Geometry: final body of the model. Coordinates: model frame, mm. A direction names the side the tool comes from. Round coordinates to 2 decimals unless told otherwise and drop trailing zeros. Loops run counter-clockwise (first coordinate to the right, second up) from the corner with the lowest first, then second, coordinate; pieces in that order, holes last. Notation, with made-up numbers: (19.5, 32.25) - (34.5, 32.25) arc R20 ccw to (34.5, 56.25) - close; hole circle Ø8 at (59, 46.25). An arc over 180 degrees is marked (long way). Answer as a JSON object with one key per item and string values. Group by question number.
Item 1: Section C-C (y = -4). Return the cut outline in (x, z), plus the area to 3 significant figures.
Item 2: Line query: line 1 (Z direction, x = 65.75, y = -2); line 2 (X direction, y = 0, z = 28.5); line 3 (Y direction, x = 66.5, z = 9.5). Output: solid intervals per line, ascending.
Item 3: Draft query along X for faces 4 (the face through (72.08, -5.04, 14.79)), 5 (the face through (67.43, 0.45, 14.87)), 6 (the face through (66, -2.95, 26)). Return one class per face: released by +X, released by -X, zero draft, split by the parting line, or undercut.
Item 4: First-contact query: pin 1 (1.5 mm diameter, centred on x = 65, z = 19.5, fed in from -Y); pin 2 (0.8 mm diameter, centred on x = 65, z = 25.5, fed in from -Y); pin 3 (0.8 mm diameter, centred on y = 0.5, z = 25.5, fed in from -X); pin 4 (4 mm diameter, centred on x = 66, y = 0, fed in from -Z). Flat tips, straight axial feed; report the tip coordinate or a pass-through.
Item 5: Section D-D (x = 65.5). Return the cut outline in (y, z).
Item 6: Reachability of faces 1 (the face through (67.4, 1.3, 27)), 2 (the face through (71.403, 3.725, 15.21)), 3 (the face through (71, 0, 4)) from +Z, -Z, +X, -X, +Y, -Y: full face, straight path, thin tool, end or side. Return the list, or none.
Item 7: Section B-B (z = 11.5). Return the cut outline in (x, y).
Item 8: Section A-A (z = 24.75). Return the cut outline in (x, y).
```python
from build123d import *

# Parameters (mm, degrees)
SKETCH_R        = 1.5
PAD_DEPTH       = 30
POCKET_DEPTH    = 30.001
FILLET_R        = 4.5
SKETCH002_W     = 5.9
SKETCH002_H     = 2.8
POCKET001_DEPTH = 71


with BuildPart() as part:
    # Sketch → Pad (new body)
    with BuildSketch(Plane.XY):
        with BuildLine():
            Line((61.848971, 4.324901), (72.822176, 5.092223))
            ThreePointArc((72.822176, -5.092223), (73, 0), (72.822176, 5.092223))
            Line((72.822176, -5.092223), (61.848971, -4.324901))
            ThreePointArc((61.848971, -4.324901), (62, 0), (61.848971, 4.324901))
        make_face()
        with Locations((66, 0)):
            Circle(SKETCH_R, mode=Mode.SUBTRACT)
    extrude(amount=PAD_DEPTH)

    # Sketch001 (on Face7 of Pad) → Pocket (cut, through all)
    with BuildSketch(Plane.XY.offset(30)):
        with BuildLine():
            ThreePointArc((71.32583, -4.987588), (71.402012, -3.742021), (71.456444, -2.495314))
            Line((69.257784, -2.418535), (71.456444, -2.495314))
            ThreePointArc((69.131189, -4.834124), (69.205027, -3.626882), (69.257784, -2.418535))
            Line((69.131189, -4.834124), (71.32583, -4.987588))
        make_face()
        with BuildLine():
            Line((69.257784, 2.418535), (71.456444, 2.495314))
            ThreePointArc((71.456444, 2.495314), (71.402012, 3.742021), (71.32583, 4.987588))
            Line((69.131189, 4.834124), (71.32583, 4.987588))
            ThreePointArc((69.257784, 2.418535), (69.205027, 3.626882), (69.131189, 4.834124))
        make_face()
    extrude(amount=-POCKET_DEPTH, mode=Mode.SUBTRACT)

    # Fillet
    fillet_edges = [part.edges().sort_by_distance(p)[0] for p in [
        (61.848971, 4.324901, 15),
        (61.848971, -4.324901, 15),
    ]]
    fillet(fillet_edges, radius=FILLET_R)

    # Sketch002 → Pocket001 (cut)
    with BuildSketch(Plane.YZ):
        with Locations((0, 25.6)):
            Rectangle(SKETCH002_W, SKETCH002_H)
        with Locations((0, 4.4)):
            Rectangle(SKETCH002_W, SKETCH002_H)
    extrude(amount=POCKET001_DEPTH, mode=Mode.SUBTRACT)


solid = part.part
```
Values:
{
 "1": {"outline": "(64.19, 0) - (69.18, 0) - (69.18, 30) - (64.19, 30) - close; (71.39, 0) - (72.89, 0) - (72.89, 30) - (71.39, 30) - close", "area": "195 mm^2"},
 "2": {"line 1": "z = 0 to 3, 5.8 to 24.2, 27 to 30", "line 2": "x = 62 to 64.5, 67.5 to 73", "line 3": "y = -4.65 to -1.41, 1.41 to 4.65"},
 "3": {"face 4": "released by -X", "face 5": "undercut", "face 6": "zero draft"},
 "4": {"pin 1": "stops at y = -4.58", "pin 2": "stops at y = -4.5", "pin 3": "stops at x = 71", "pin 4": "stops at z = 0"},
 "5": {"outline": "(-4.53, 0) - (-1.41, 0) - (-1.41, 3) - (-2.95, 3) - (-2.95, 5.8) - (-1.41, 5.8) - (-1.41, 24.2) - (-2.95, 24.2) - (-2.95, 27) - (-1.41, 27) - (-1.41, 30) - (-4.53, 30) - close; (1.41, 0) - (4.53, 0) - (4.53, 30) - (1.41, 30) - (1.41, 27) - (2.95, 27) - (2.95, 24.2) - (1.41, 24.2) - (1.41, 5.8) - (2.95, 5.8) - (2.95, 3) - (1.41, 3) - close"},
 "6": {"face 1": "-X", "face 2": "+Z, -Z", "face 3": "-X, +Y, -Y"},
 "7": {"outline": "(62, -0.13) arc R4.5 ccw to (66.19, -4.63) - (69.13, -4.83) arc R69.3 ccw to (69.26, -2.42) - (71.46, -2.5) arc R71.5 cw to (71.33, -4.99) - (72.82, -5.09) arc R73 ccw to (72.82, 5.09) - (71.33, 4.99) arc R71.5 cw to (71.46, 2.5) - (69.26, 2.42) arc R69.3 ccw to (69.13, 4.83) - (66.19, 4.63) arc R4.5 ccw to (62, 0.13) arc R62 cw to start; hole circle Ø3 at (66, 0)"},
 "8": {"outline": "(62.99, -2.95) arc R4.5 ccw to (66.19, -4.63) - (69.13, -4.83) arc R69.3 ccw to (69.24, -2.95) - close; (62.99, 2.95) - (69.24, 2.95) arc R69.3 ccw to (69.13, 4.83) - (66.19, 4.63) arc R4.5 ccw to start; (71, -2.48) - (71.46, -2.5) arc R71.5 cw to (71.33, -4.99) - (72.82, -5.09) arc R73 ccw to (72.82, 5.09) - (71.33, 4.99) arc R71.5 cw to (71.46, 2.5) - (71, 2.48) - close"}
}
